```python
from build123d import *

# Parameters (mm, degrees)
F1_DEPTH = 750
F2_R     = 2.5
F3_R     = 3
F4_R     = 5
F5_R     = 5.5


with BuildPart() as f1:
    # F0 (on Front) → F1 (new body, symmetric)
    with BuildSketch(Plane.XZ):
        Polygon((-1, -20.571158), (-1.5, -20.571158), (-1.5, -32.527116), (-21, -35.965492), (-21, -56.274024), (0, -52.571158), (0, 52.571158), (-21, 56.274024), (-21, 35.965492), (-1.5, 32.527116), (-1.5, 20.571158), (-1, 20.571158), (-1, 32.946666), (-20.5, 36.385042), (-20.5, 55.678148), (-0.5, 52.151608), (-0.5, -52.151608), (-20.5, -55.678148), (-20.5, -36.385042), (-1, -32.946666), align=None)
    extrude(amount=F1_DEPTH, both=True)

    # F2
    f2_edges = [f1.edges().sort_by_distance(p)[0] for p in [
        (-0.5, 0, 52.151608),
        (-20.5, 0, 36.385042),
        (-20.5, 0, 55.678148),
        (-20.5, 0, -36.385042),
        (-0.5, 0, -52.151608),
        (-20.5, 0, -55.678148),
    ]]
    fillet(f2_edges, radius=F2_R)

    # F3
    f3_edges = [f1.edges().sort_by_distance(p)[0] for p in [
        (0, 0, 52.571158),
        (-21, 0, 35.965492),
        (-21, 0, 56.274024),
        (-21, 0, -35.965492),
        (-21, 0, -56.274024),
        (0, 0, -52.571158),
    ]]
    fillet(f3_edges, radius=F3_R)

    # F4
    f4_edges = [f1.edges().sort_by_distance(p)[0] for p in [
        (-1.5, 0, 32.527116),
        (-1.5, 0, -32.527116),
    ]]
    fillet(f4_edges, radius=F4_R)

    # F5
    f5_edges = [f1.edges().sort_by_distance(p)[0] for p in [
        (-1, 0, -32.946666),
        (-1, 0, 32.946666),
    ]]
    fillet(f5_edges, radius=F5_R)


solid = f1.part
```
Geometry: final body of the model. Coordinates: model frame, mm. Coordinates: 2 decimals unless noted, no trailing zeros. Order: outer loops, then holes, each group sorted by start corner. A loop starts at its lowest first (then second) coordinate and runs counter-clockwise, first axis right, second up. Notation, with made-up numbers: (65, 81.5) - (106, 81.5) arc R24 cw to (106, 107.5) - close; hole circle Ø11 at (20, 70.5). An arc over 180 degrees is marked (long way). Return JSON: item names as keys, results as strings. Group by question number.
1. Material intervals for line 1 along Z through (x, y) = (-17.75, -430.5); line 2 along X through (y, z) = (327.5, 45); line 3 along Z through (x, y) = (-4.5, 474.5), sorted ascending. Write a range as [from, to].
2. Cut plane B-B (z = 4). Output: boundary loops of the cut face in (x, y), plus the area to 3 significant figures.
3. Cut plane A-A (x = -10). Output: boundary loops of the cut face in (y, z).
4. Pull-direction query (X, two-part tool) for faces 1 (the face through (0, -10, -1)), 2 (the face through (-0.5, -10, 1)); classes: pulls with the +X half, pulls with the -X half, needs draft (parallel to the pull), parting line crosses it, or undercut.
5. Pin query (flat end, axial travel): pin 1 (0.6 mm diameter, centred on x = -1.5, y = 203, fed in from +Z); pin 2 (1 mm diameter, centred on x = -2.5, y = 441, fed in from +Z); pin 3 (8.5 mm diameter, centred on y = -226, z = 25, fed in from -X). Return the tip coordinate at first contact, or that it passes through.
Resolved:
{
 "1": {"line 1": "z = [-55.69, -55.19], [-35.9, -35.39], [35.39, 35.9], [55.19, 55.69]", "line 2": "x = [-21, -20.5], [-0.5, 0]", "line 3": "z = [-53.36, -52.86], [-33.46, -32.91], [32.91, 33.46], [52.86, 53.36]"},
 "2": {"outline": "(-0.5, -750) - (0, -750) - (0, 750) - (-0.5, 750) - close", "area": "750 mm²"},
 "3": {"outline": "(-750, -54.33) - (750, -54.33) - (750, -53.83) - (-750, -53.83) - close; (-750, -34.53) - (750, -34.53) - (750, -34.03) - (-750, -34.03) - close; (-750, 34.03) - (750, 34.03) - (750, 34.53) - (-750, 34.53) - close; (-750, 53.83) - (750, 53.83) - (750, 54.33) - (-750, 54.33) - close"},
 "4": {"face 1": "pulls with the +X half", "face 2": "undercut"},
 "5": {"pin 1": "stops at z = 52.8", "pin 2": "stops at z = 53.1", "pin 3": "stops at x = -1.59"}
}
